from build123d import *

# Parameters (mm, degrees)
F1_DEPTH = 6.35
F2_R     = 3.81
F3_DEPTH = 3.81


with BuildPart() as f1:
    # F0 (on Front) → F1 (new body)
    with BuildSketch(Plane.XZ):
        with BuildLine():
            Line((-23.164801, 34.290001), (-17.347254, 19.659236))
            ThreePointArc((-17.347254, 19.659236), (-24.492601, 9.355494), (-26.036071, -3.088009))
            Line((-26.036071, -3.088009), (-34.442399, -4.113362))
            Line((-34.442399, -4.113362), (-25.89388, -4.113362))
            ThreePointArc((-25.89388, -4.113362), (-25.638984, -5.482267), (-25.311773, -6.835709))
            Line((-25.311773, -6.835709), (-35.966402, -8.135295))
            Line((-35.966402, -8.135295), (-24.924481, -8.135295))
            ThreePointArc((-24.924481, -8.135295), (-24.14935, -10.208901), (-23.202056, -12.209725))
            Line((-23.202056, -12.209725), (-34.442401, -13.489514))
            Line((-34.442401, -13.489514), (-22.482121, -13.489514))
            ThreePointArc((-22.482121, -13.489514), (-19.455276, -17.575694), (-15.696574, -21.000722))
            Line((-15.696574, -21.000722), (-40.337007, -21.000722))
            Line((-40.337007, -21.000722), (-42.792861, -15.918796))
            Line((-42.792861, -15.918796), (-48.1584, -23.711554))
            Line((-48.1584, -23.711554), (-11.188163, -23.711554))
            ThreePointArc((-11.188163, -23.711554), (8.251092, -24.886387), (23.137988, -12.330704))
            Line((23.137988, -12.330704), (36.880807, -12.330704))
            Line((36.880807, -12.330704), (23.661428, -11.293785))
            ThreePointArc((23.661428, -11.293785), (24.231756, -10.011733), (24.732677, -8.701004))
            Line((24.732677, -8.701004), (35.052002, -8.701004))
            Line((35.052002, -8.701004), (24.898263, -8.215185))
            ThreePointArc((24.898263, -8.215185), (25.442691, -6.331056), (25.844756, -4.411501))
            Line((25.844756, -4.411501), (35.356801, -4.411501))
            Line((35.356801, -4.411501), (25.925817, -3.907015))
            ThreePointArc((25.925817, -3.907015), (24.780888, 8.562731), (17.9832, 19.079237))
            Line((17.9832, 19.079237), (17.9832, 34.5948))
            Line((17.9832, 34.5948), (6.210996, 25.472265))
            ThreePointArc((6.210996, 25.472265), (-1.012157, 26.199014), (-8.15771, 24.917153))
            Line((-8.15771, 24.917153), (-23.164801, 34.290001))
        make_face()
    extrude(amount=F1_DEPTH)

    # F2 (on face) → F3 (cut)
    with BuildSketch(Plane.XZ.offset(6.35)):
        with Locations((8.507902, 10.2108)):
            Circle(F2_R)
        with Locations((-14.601506, 9.602658)):
            Circle(F2_R)
        with BuildLine():
            ThreePointArc((-6.682666, -13.016536), (-15.195966, -8.000344), (-20.67365, 0.223613))
            ThreePointArc((-20.67365, 0.223613), (0, -20.674859), (20.67365, 0.223613))
            ThreePointArc((20.67365, 0.223613), (14.449008, -8.675643), (4.737722, -13.537109))
            Line((4.737722, -13.537109), (5.596831, -17.513046))
            Line((5.596831, -17.513046), (1.264551, -18.449153))
            Line((1.264551, -18.449153), (0.280041, -13.892863))
            Line((0.280041, -13.892863), (-1.722237, -13.983534))
            ThreePointArc((-1.722237, -13.983534), (-2.586056, -13.898947), (-3.445889, -13.780519))
            Line((-3.445889, -13.780519), (-5.150155, -18.254217))
            Line((-5.150155, -18.254217), (-9.041306, -16.771873))
            Line((-9.041306, -16.771873), (-6.682666, -13.016536))
        make_face()
    extrude(amount=-F3_DEPTH, mode=Mode.SUBTRACT)


solid = f1.part
Design review of the part built by this model. Coordinates are the model's own, in mm. A direction names the side the tool comes from. Round coordinates to 2 decimals unless told otherwise and drop trailing zeros. Write each loop counter-clockwise with the first axis right and the second up, starting at its lowest first coordinate (ties: lowest second). Pieces come first, ordered by that corner, then holes. Notation, with made-up numbers: (-17, 36) -> (42, 36) arc R18 cw to (42, 70) -> close; hole circle Ø6 at (34.25, -7). An arc over 180 degrees is marked (long way). One line per question, with ' | ' between items.
(1) Machinability: for faces 1 (the flat face through (-30, -3, -23.712)), 2 (the flat face through (-15, -2.54, 10)), 3 (the flat face through (12.18, -3.13, 30.1)), 4 (the flat face through (30.36, -3.13, -11.82)), which of the approach directions +Z, -Z, +X, -X, +Y, -Y give a long, thin tool a straight path to every point of the face, cutting with its end or side? Answer none if there is none.
Result sheet:
face 1: -Z, -X, +Y, -Y | face 2: -Y | face 3: +Z, +Y, -Y | face 4: +X, +Y, -Y
(2) Insertion check: P1, Ø1.9, axis at x = -29, y = -4, coming from the -Z side; P2, Ø3, axis at x = 31, y = -3, coming from the -Z side; P3, Ø2, axis at x = 5, y = -3.5, coming from the -Z side; P4, Ø1.5, axis at x = 21, z = 17.5, coming from the +Y side. Each pin has a flat end and moves straight along its axis. Give the tip position at first contact, or say it passes through.
Result sheet:
P1: z = -23.71 | P2: z = -12.33 | P3: z = -25.91 | P4: through
(3) Take a section at B-B, the plane x = -28. State the section outline as (y, z) points, and give its area (3 significant figures).
Result sheet:
outline: (-6.35, -23.71) -> (0, -23.71) -> (0, -21) -> (-6.35, -21) -> close; (-6.35, -13.49) -> (0, -13.49) -> (0, -12.76) -> (-6.35, -12.76) -> close; (-6.35, -8.14) -> (0, -8.14) -> (0, -7.16) -> (-6.35, -7.16) -> close; (-6.35, -4.11) -> (0, -4.11) -> (0, -3.33) -> (-6.35, -3.33) -> close | area: 33.0 mm2
(4) Wall thickness on line 1 (X direction, y = -5.75, z = -3); line 2 (Z direction, x = -30, y = -0.5); line 3 (Z direction, x = -38.5, y = -3): over which ranges is each line inside the solid? List them lowest first. Write a range as [from, to].
Result sheet:
line 1: [-26.05, -20.46], [-19.14, 19.14], [20.46, 26.05] | line 2: [-23.71, -21], [-13.49, -12.98], [-8.14, -7.41], [-4.11, -3.57] | line 3: [-23.71, -21]
(5) Draft analysis for pull direction Z (two halves, no side actions). For faces 5 (the flat face through (31, -3, -4.412)), 6 (the cylindrical face through (-0.91, -3.131, 26.203)), 7 (the flat face through (17.983, -3, 27)), state which applies: released by +Z, released by -Z, zero draft, split by the parting line, or undercut.
Result sheet:
face 5: undercut | face 6: released by +Z | face 7: zero draft
(6) Take a section at D-D, the plane y = -5.5. State how many separate pieces and enclosed holes the cut face has, and give its area (3 significant figures).
Result sheet:
separate pieces: 1 | enclosed holes: 3 | area: 2,150 mm2
(7) Take a section at C-C, the plane x = 17. State the section outline as (y, z) points, and give its area (3 significant figures).
Result sheet:
outline: (-6.35, -19.96) -> (0, -19.96) -> (0, 33.83) -> (-6.35, 33.83) -> (-6.35, -6.08) -> (-2.54, -6.08) -> (-2.54, -11.77) -> (-6.35, -11.77) -> close | area: 320 mm2
